from build123d import *

# Parameters (mm, degrees)
SKETCH_1_W      = 70
SKETCH_1_H      = 22.5
EXTRUDE_1_DEPTH = 9.5
SKETCH_2_R      = 2.5
EXTRUDE_2_DEPTH = 8.5


with BuildPart() as part:
    # 草图1 → 凸台-拉伸1 (new, symmetric)
    with BuildSketch(Plane.XY):
        Rectangle(SKETCH_1_W, SKETCH_1_H)
    extrude(amount=EXTRUDE_1_DEPTH, both=True)

    # 草图2 → 凸台-拉伸2 (add)
    with BuildSketch(Plane.XY.offset(9.5)):
        with Locations(Location((25.865182866, 0, 0), (0, 0, 180))):
            Circle(SKETCH_2_R)
    extrude_2 = extrude(amount=EXTRUDE_2_DEPTH)

    # 镜向1: 凸台-拉伸2 across plane
    add(extrude_2.mirror(Plane.XY))


solid = part.part
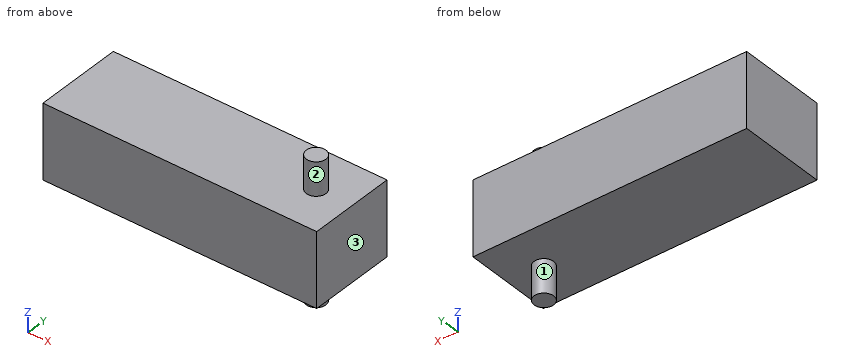
Work out the finished part from the listing and answer in its coordinate system (mm). Face numbers are marked on the shaded views. A direction names the side the tool comes from. Give positions to 0.01 mm unless a question says otherwise; leave off trailing zeros. Order: outer loops, then holes, each group sorted by start corner. A loop starts at its lowest first (then second) coordinate and runs counter-clockwise, first axis right, second up. Notation, with made-up numbers: M 27.5,-36 L 45.5,-36 A20 ccw 45.5,-6 Z; hole C 59,-18 d1. An arc over 180 degrees is marked long. Return JSON: item names as keys, results as strings.
Q1. Which of the six approach directions +Z, -Z, +X, -X, +Y, -Y give full straight-line access (tool end or side, diameter ignored) to the marked faces 1, 2 and 3?
Answer below:
{"face 1": "-Z", "face 2": "+Z", "face 3": "+Z, -Z, +X, +Y, -Y"}
Q2. Each of these flat-tipped pins is pushed along its axis until it touches: pin 1 (8 mm diameter, centred on x = 18, z = -14, fed in from +Y); pin 2 (11 mm diameter, centred on x = -12.5, y = 3, fed in from +Z); pin 3 (12 mm diameter, centred on x = -19.5, y = 8, fed in from -Z). Where does it stop, or does it pass through?
Answer below:
{"pin 1": "passes through", "pin 2": "stops at z = 9.5", "pin 3": "stops at z = -9.5"}
Q3. Find the intervals of material crossed by line 1 along Z through (x, y) = (21.5, 1.5); line 2 along X through (y, z) = (-0.75, 16); line 3 along X through (y, z) = (2, 14.5), in increasing order. Write a range as [from, to].
Answer below:
{"line 1": "z = [-9.5, 9.5]", "line 2": "x = [23.48, 28.25]", "line 3": "x = [24.37, 27.37]"}
Q4. Find section C-C, the plane y = -4.25. Write down the section's boundary in (x, z).
Answer below:
{"outline": "M -35,-9.5 L 35,-9.5 L 35,9.5 L -35,9.5 Z"}
Q5. Find section A-A, the plane y = 0. Write down the section's boundary in (x, z), and give its area (4 significant figures).
Answer below:
{"outline": "M -35,-9.5 L 23.37,-9.5 L 23.37,-18 L 28.37,-18 L 28.37,-9.5 L 35,-9.5 L 35,9.5 L 28.37,9.5 L 28.37,18 L 23.37,18 L 23.37,9.5 L -35,9.5 Z", "area": "1,415 mm^2"}
Q6. Find section B-B, the plane x = 31. Write down the section's boundary in (y, z), and give its area (4 significant figures).
Answer below:
{"outline": "M -11.25,-9.5 L 11.25,-9.5 L 11.25,9.5 L -11.25,9.5 Z", "area": "427.5 mm^2"}
